Here's how the part is built. I have some questions about the finished solid (model axes, mm). A direction names the side the tool comes from. Round coordinates to 2 decimals unless told otherwise and drop trailing zeros. Order: outer loops, then holes, each group sorted by start corner. A loop starts at its lowest first (then second) coordinate and runs counter-clockwise, first axis right, second up. Notation, with made-up numbers: (86, -27) - (104, -27) arc R11 ccw to (104, -6) - close; hole circle Ø11 at (-18, 60). An arc over 180 degrees is marked (long way). One line per item, written item: value.
Autodesk Inventor part; units mm, degrees
ref_plane "YZ Plane" through (0, 0, 0) normal (1, 0, 0) x (0, 1, 0)
ref_plane "XZ Plane" through (0, 0, 0) normal (0, 1, 0) x (-1, 0, 0)
ref_plane "XY Plane" through (0, 0, 0) normal (0, 0, 1) x (1, 0, 0)
sketch "Sketch1" plane through (0, 0, 0) normal (0, 0, 1) x (1, 0, 0)
  circle A0 centre (5.0032, 3.2866) radius 1.82
  point P0 (0, 0)
  dimension "d0" = 3.64
extrude "Extrusion1" add sketch "Sketch1" along normal blind 2
sketch "Sketch2" plane through (5.0032, 3.2866, 2) normal (0, 0, 1) x (1, 0, 0)
  circle A0 centre (0, 0) radius 0.75
  point P0 (-5.0032, -3.2866)
  dimension "d3" = 1.5
extrude "Extrusion2" cut sketch "Sketch2" against normal through all
sketch "Sketch3" plane through (5.0032, 3.2866, 2) normal (0, 0, 1) x (1, 0, 0)
  line L0 (0, -1.82) -> (0, -0.682) construction
  line L1 (-1.6874, -0.682) -> (-1.4874, -0.682)
  circle A0 centre (0, 0) radius 1.82
  circle A1 centre (0, 0) radius 1.6363
  line L2 (0, 1.6363) -> (0, 1.82)
  point P0 (-5.0032, -3.2866)
  point P1 (0.02, 0)
  dimension "d6" = 1.138
  dimension "d7" = 0.2
extrude "Extrusion3" cut sketch "Sketch3" against normal through all contours A0 L2 A1 L1 picked at (-0.267, 1.7273)
sketch "Sketch5" plane through (0, 0, 0) normal (0, 0, -1) x (-1, 0, 0)
  line L0 (-3.3158, 2.6046) -> (-3.5158, 2.6046)
  arc A0 (-3.5158, 2.6046) -> (-5.0032, 4.9229) centre (-5.0032, 3.2866) ccw
  line L1 (-5.0032, 4.9229) -> (-5.0032, 5.1066)
  arc A1 (-5.0032, 5.1066) -> (-3.3158, 2.6046) centre (-5.0032, 3.2866) ccw
  circle A2 centre (-5.0032, 3.2866) radius 0.75
  line L2 (-3.5158, 2.6046) -> (-3.5158, 2.2377) construction
  arc A3 (-5.0032, 5.1066) -> (-3.3158, 2.6046) centre (-5.0032, 3.2866) ccw
  line L3 (-3.5158, 3.9686) -> (-3.5158, 0)
  line L4 (-3.5158, 0) -> (0.9842, 0)
  line L5 (0.9842, 0) -> (0.9842, 3.9686)
  line L6 (0.9842, 3.9686) -> (-3.5158, 3.9686)
  arc A4 (0.9842, 0) -> (0.9842, 3.9686) centre (0.3524, 1.9843) ccw
  point P0 (0, 0)
  dimension "d18" = 4.5
extrude "Extrusion6" add sketch "Sketch5" against normal up to surface (2 mm away) contours L0 A0 L6 L5 L4 L3 A1 | A4 L5
properties material "Liga de Nickel-Copper 400"
Q1. If we section it at A-A, the plane y = 3.5: Please give me the cut outline in (x, z).
Results list:
outline: (-1.78, 0) - (4.28, 0) - (4.28, 2) - (-1.78, 2) - close; (5.72, 0) - (6.81, 0) - (6.81, 2) - (5.72, 2) - close
Q2. We'd pull the mould along X, two halves only. Please class faces 1 (the cylindrical face through (6.642, 2.496, 0.986)), 2 (the cylindrical face through (-2.435, 1.947, 0.986)), 3 (the flat face through (2, 3, 2)): released by +X, released by -X, zero draft, split by the parting line, or undercut.
Results list:
face 1: undercut
face 2: released by -X
face 3: zero draft
Q3. If we section it at D-D, the plane y = 2.7: Please give me the cut outline in (x, z), then the cut area to 3 significant figures.
Results list:
outline: (-2.31, 0) - (4.54, 0) - (4.54, 2) - (-2.31, 2) - close; (5.47, 0) - (6.73, 0) - (6.73, 2) - (5.47, 2) - close
area: 16.2 mm²
Q4. If I drill on line 1 along Y through (x, z) = (-0.25, 1); line 2 along X through (y, z) = (3.45, 1.35); line 3 along X through (y, z) = (2.9, 0.2), over which ranges is the centre line in solid material (lowest first)?
Results list:
line 1: 0 to 3.97
line 2: -1.83 to 4.27, 5.74 to 6.82
line 3: -2.22 to 4.36, 5.65 to 6.78
Q5. Which directions (+Z, -Z, +X, -X, +Y, -Y) give clear straight access to the entire face, cutting with the end or side of a thin tool? Please do faces 4 (the flat face through (3.516, 1, 1)), 5 (the flat face through (1, 3.969, 1)), 6 (the flat face through (1, 0, 1)).
Results list:
face 4: +Z, -Z, -Y
face 5: +Z, -Z, -X, +Y
face 6: +Z, -Z, +X, -X, -Y
Q6. If we section it at C-C, the plane x = 0.75: Please give me the cut outline in (y, z), then the cut area to 3 significant figures.
Results list:
outline: (0, 0) - (3.97, 0) - (3.97, 2) - (0, 2) - close
area: 7.94 mm²
Q7. Will these pins go through, and if not, where does the flat tip stop? pin 1 (0.6 mm diameter, centred on x = 2, z = 1, fed in from +Y); pin 2 (2 mm diameter, centred on x = 5, y = 3.29, fed in from +Z).
Results list:
pin 1: y = 3.97
pin 2: z = 2
Q8. If we section it at B-B, the plane z = 0.8: Please give me the cut outline in (x, y), then the cut area to 3 significant figures.
Results list:
outline: (-0.98, 0) - (3.52, 0) - (3.52, 2.24) arc R1.82 ccw (long way) to (5, 5.11) - (5, 4.92) arc R1.64 ccw to (3.52, 3.97) - (-0.98, 3.97) arc R2.08 ccw to start; hole circle Ø1.5 at (5, 3.29)
area: 29.9 mm²
